from build123d import *

# Parameters (mm, degrees)
F0_R     = 9.5
F1_DEPTH = 5


# Not quite as in the source:
# - a feature names something its author has since deleted; it is built from what else it names


with BuildPart() as f1:
    # F0 (on Top) → F1 (new body)
    with BuildSketch(Plane.XY):
        with BuildLine():
            ThreePointArc((-13.665469042, -3.0319204432), (-13.3159762762, 4.3418317), (-9.2645390994, 10.5127491897))
            ThreePointArc((-9.2645390994, 10.5127491897), (-11.4998669549, 9.7726015122), (-13.5809814233, 10.8741784618))
            Line((-13.5809814233, 10.8741784618), (-20.506494271, 19.426474585))
            ThreePointArc((-20.506494271, 19.426474585), (-29.538567909, 20.601795911), (-32.0861364699, 11.8571044442))
            ThreePointArc((-32.0861364699, 11.8571044442), (-32.0062029861, 10.4146544851), (-32.9187213461, 9.2946716776))
            ThreePointArc((-32.9187213461, 9.2946716776), (-35.997695766, 0.7226444411), (-27.9997581563, -3.6354203143))
            Line((-27.9997581563, -3.6354203143), (-17.3699870332, -0.7871817262))
            ThreePointArc((-17.3699870332, -0.7871817262), (-15.0388393758, -1.1192356462), (-13.665469042, -3.0319204432))
        make_face()
        Polygon((-28.6916231536, 13.1985965214), (-21.5082094645, 14.7254782362), (-16.5941842664, 9.267900353), (-18.8635727573, 2.2834407549), (-26.0469864464, 0.7565590401), (-30.9610116446, 6.2141369233), align=None, mode=Mode.SUBTRACT)
        with BuildLine():
            ThreePointArc((9.2621690031, 10.5127491897), (8.227808484, 11.3418317), (7.1196691813, 12.0693664265))
            ThreePointArc((7.1196691813, 12.0693664265), (-0.0011850481, 14.0155937788), (-7.1220392775, 12.0693664265))
            ThreePointArc((-7.1220392775, 12.0693664265), (-8.2301785802, 11.3418317), (-9.2645390994, 10.5127491897))
            ThreePointArc((-9.2645390994, 10.5127491897), (-13.3159762762, 4.3418317), (-13.665469042, -3.0319204432))
            ThreePointArc((-13.665469042, -3.0319204432), (-13.3159762762, -4.3106441425), (-12.847106931, -5.5505800398))
            ThreePointArc((-12.847106931, -5.5505800398), (-8.2301785802, -11.3106441425), (-1.3253227589, -13.9216462393))
            ThreePointArc((-1.3253227589, -13.9216462393), (-0.0011850481, -13.9844062212), (1.3229526627, -13.9216462393))
            ThreePointArc((1.3229526627, -13.9216462393), (8.227808484, -11.3106441425), (12.8447368348, -5.5505800398))
            ThreePointArc((12.8447368348, -5.5505800398), (13.31360618, -4.3106441425), (13.6630989458, -3.0319204432))
            ThreePointArc((13.6630989458, -3.0319204432), (13.9146328566, -1.5173811207), (13.9988149519, 0.0155937788))
            ThreePointArc((13.9988149519, 0.0155937788), (12.7598289539, 5.7737637694), (9.2621690031, 10.5127491897))
        make_face()
        Circle(F0_R, mode=Mode.SUBTRACT)
        with BuildLine():
            ThreePointArc((-1.3253227589, -13.9216462393), (-8.2301785802, -11.3106441425), (-12.847106931, -5.5505800398))
            ThreePointArc((-12.847106931, -5.5505800398), (-12.8339389546, -7.9052213736), (-14.5247006287, -9.5440728519))
            Line((-14.5247006287, -9.5440728519), (-24.7985187507, -13.4878221314))
            ThreePointArc((-24.7985187507, -13.4878221314), (-28.7073800051, -21.7146403569), (-21.1779261823, -26.8397803113))
            ThreePointArc((-21.1779261823, -26.8397803113), (-19.7813739443, -27.2095006015), (-18.998190678, -28.4234508549))
            ThreePointArc((-18.998190678, -28.4234508549), (-11.7971637379, -34.0006316328), (-5.1808992125, -27.7408570242))
            Line((-5.1808992125, -27.7408570242), (-4.6049551583, -16.7511898031))
            ThreePointArc((-4.6049551583, -16.7511898031), (-3.5687888714, -14.6367469374), (-1.3253227589, -13.9216462393))
        make_face()
        Polygon((-21.4047986615, -23.1968624525), (-20.6371525584, -15.8931976559), (-13.9281702523, -12.906166284), (-7.9868340493, -17.2227997087), (-8.7544801524, -24.5264645053), (-15.4634624585, -27.5134958771), align=None, mode=Mode.SUBTRACT)
        with BuildLine():
            ThreePointArc((7.1196691813, 12.0693664265), (5.7249926142, 13.9665713389), (6.1295548123, 16.2862348132))
            Line((6.1295548123, 16.2862348132), (12.1231706049, 25.5155937788))
            ThreePointArc((12.1231706049, 25.5155937788), (10.4499033622, 34.4688005315), (1.34596558, 34.1894239382))
            ThreePointArc((1.34596558, 34.1894239382), (-0.0011850481, 33.6676611266), (-1.3483356762, 34.1894239382))
            ThreePointArc((-1.3483356762, 34.1894239382), (-10.4522734584, 34.4688005315), (-12.1255407011, 25.5155937788))
            Line((-12.1255407011, 25.5155937788), (-6.1319249085, 16.2862348132))
            ThreePointArc((-6.1319249085, 16.2862348132), (-5.7273627104, 13.9665713389), (-7.1220392775, 12.0693664265))
            ThreePointArc((-7.1220392775, 12.0693664265), (-0.0011850481, 14.0155937788), (7.1196691813, 12.0693664265))
        make_face()
        Polygon((-7.3450804722, 25.0155937788), (-3.6731327602, 31.3755937788), (3.6707626639, 31.3755937788), (7.342710376, 25.0155937788), (3.6707626639, 18.6555937788), (-3.6731327602, 18.6555937788), align=None, mode=Mode.SUBTRACT)
        with BuildLine():
            ThreePointArc((14.5223305325, -9.5440728519), (12.8315688584, -7.9052213736), (12.8447368348, -5.5505800398))
            ThreePointArc((12.8447368348, -5.5505800398), (8.227808484, -11.3106441425), (1.3229526627, -13.9216462393))
            ThreePointArc((1.3229526627, -13.9216462393), (3.5664187752, -14.6367469374), (4.6025850621, -16.7511898031))
            Line((4.6025850621, -16.7511898031), (5.1785291162, -27.7408570242))
            ThreePointArc((5.1785291162, -27.7408570242), (11.7947936417, -34.0006316328), (18.9958205818, -28.4234508549))
            ThreePointArc((18.9958205818, -28.4234508549), (19.7790038481, -27.2095006015), (21.1755560861, -26.8397803113))
            ThreePointArc((21.1755560861, -26.8397803113), (28.7050099089, -21.7146403569), (24.7961486545, -13.4878221314))
            Line((24.7961486545, -13.4878221314), (14.5223305325, -9.5440728519))
        make_face()
        Polygon((7.9844639531, -17.2227997087), (13.9258001561, -12.906166284), (20.6347824622, -15.8931976559), (21.4024285653, -23.1968624525), (15.4610923623, -27.5134958771), (8.7521100562, -24.5264645053), align=None, mode=Mode.SUBTRACT)
        with BuildLine():
            ThreePointArc((13.5786113271, 10.8741784618), (11.4974968587, 9.7726015122), (9.2621690031, 10.5127491897))
            ThreePointArc((9.2621690031, 10.5127491897), (12.7598289539, 5.7737637694), (13.9988149519, 0.0155937788))
            ThreePointArc((13.9988149519, 0.0155937788), (13.9146328566, -1.5173811207), (13.6630989458, -3.0319204432))
            ThreePointArc((13.6630989458, -3.0319204432), (15.0364692796, -1.1192356462), (17.367616937, -0.7871817262))
            Line((17.367616937, -0.7871817262), (27.99738806, -3.6354203143))
            ThreePointArc((27.99738806, -3.6354203143), (35.9953256698, 0.7226444411), (32.9163512498, 9.2946716776))
            ThreePointArc((32.9163512498, 9.2946716776), (32.0038328898, 10.4146544851), (32.0837663737, 11.8571044442))
            ThreePointArc((32.0837663737, 11.8571044442), (29.5361978128, 20.601795911), (20.5041241748, 19.426474585))
            Line((20.5041241748, 19.426474585), (13.5786113271, 10.8741784618))
        make_face()
        Polygon((18.8612026611, 2.2834407549), (16.5918141702, 9.267900353), (21.5058393683, 14.7254782362), (28.6892530574, 13.1985965214), (30.9586415484, 6.2141369233), (26.0446163502, 0.7565590401), align=None, mode=Mode.SUBTRACT)
    extrude(amount=F1_DEPTH)


solid = f1.part
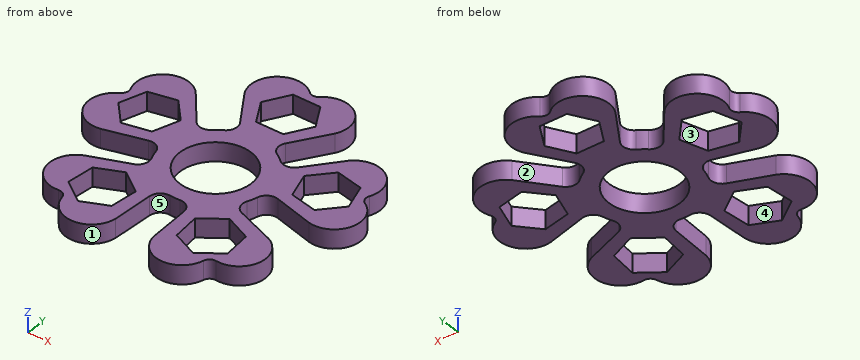
For this review, take the finished solid that the model builds, in its own axes (mm). Face numbers are marked on the shaded views. A direction names the side the tool comes from. Coordinates: 2 decimals unless noted, no trailing zeros. Loops run counter-clockwise (first coordinate to the right, second up) from the corner with the lowest first, then second, coordinate; pieces in that order, holes last. Notation, with made-up numbers: (78.5, 87.5) - (106.5, 87.5) arc R18 ccw to (106.5, 120.5) - close; hole circle Ø9 at (89.5, 75.25). An arc over 180 degrees is marked (long way). Return JSON: item names as keys, results as strings.
Item 1: Take a section at B-B (y = -2). Give the boundary of the cut face in (x, z).
Determined:
{"outline": "(-34.13, 0) - (-21.9, 0) - (-21.9, 5) - (-34.13, 5) - close; (-14.11, 0) - (-9.29, 0) - (-9.29, 5) - (-14.11, 5) - close; (9.29, 0) - (14.11, 0) - (14.11, 5) - (9.29, 5) - close; (21.89, 0) - (34.13, 0) - (34.13, 5) - (21.89, 5) - close"}
Item 2: For the marked faces 4 and 5, list the 3-axis set-ups (+Z, -Z, +X, -X, +Y, -Y) from which the entire face can be reached by the end or side of a thin tool; tool diameter is ignored.
Determined:
{"face 4": "+Z, -Z", "face 5": "+Z, -Z, -Y"}
Item 3: Take a section at D-D (y = 7.5). Give the boundary of the cut face in (x, z), then the cut area to 3 significant figures.
Determined:
{"outline": "(-34.99, 0) - (-30.54, 0) - (-30.54, 5) - (-34.99, 5) - close; (-17.17, 0) - (-5.83, 0) - (-5.83, 5) - (-17.17, 5) - close; (5.83, 0) - (17.17, 0) - (17.17, 5) - (5.83, 5) - close; (30.54, 0) - (34.99, 0) - (34.99, 5) - (30.54, 5) - close", "area": "158 mm2"}
Item 4: Take a section at C-C (z = 3.95). State how many separate pieces and enclosed holes the cut face has, then the cut area to 3 significant figures.
Determined:
{"separate pieces": "1", "enclosed holes": "6", "area": "1,830 mm2"}
Item 5: Take a section at A-A (x = 0). Give the boundary of the cut face in (y, z).
Determined:
{"outline": "(-13.98, 0) - (-9.5, 0) - (-9.5, 5) - (-13.98, 5) - close; (9.5, 0) - (18.66, 0) - (18.66, 5) - (9.5, 5) - close; (31.38, 0) - (33.67, 0) - (33.67, 5) - (31.38, 5) - close"}
Item 6: Insertion check: pin 1 (1.5 mm diameter, centred on y = 19, z = 3, fed in from +X); pin 2 (1.5 mm diameter, centred on x = -20.5, z = 3, fed in from +Y); pin 3 (3 mm diameter, centred on x = -15.5, y = -14.5, fed in from -Z); pin 4 (1.5 mm diameter, centred on x = 2, z = 3, fed in from +Y). Each pin has a flat end and moves straight along its axis. Give the tip position at first contact, or say it passes through.
Determined:
{"pin 1": "stops at x = 31.76", "pin 2": "stops at y = 20.14", "pin 3": "stops at z = 0", "pin 4": "stops at y = 35.18"}
Item 7: Mouldability with a two-part tool opening along Y and no side actions: class the marked faces 1, 2 and 3 as pulls with the +Y half, pulls with the -Y half, needs draft (parallel to the pull), parting line crosses it, or undercut.
Determined:
{"face 1": "pulls with the -Y half", "face 2": "pulls with the +Y half", "face 3": "undercut"}
Item 8: For line 1 (Y direction, x = 0, z = 2.35); line 2 (Y direction, x = -16.5, z = 2.1); line 3 (X direction, y = -15, z = 1.75), list the stretches that pass through material, from the lowest coordinate up.
Determined:
{"line 1": "y = -13.98 to -9.5, 9.5 to 18.66, 31.38 to 33.67", "line 2": "y = -32.49 to -26.76, -14.05 to -10.3, -0.69 to 14.48", "line 3": "x = -26.97 to -18.63, -11.05 to -3.92, 3.92 to 11.04, 18.63 to 26.96"}
